Check sheet for the modelled part. Datum: model origin and axes. Units: mm. Face numbers are marked on the shaded views. A direction names the side the tool comes from. Coordinates: 2 decimals unless noted, no trailing zeros. Order: outer loops, then holes, each group sorted by start corner. A loop starts at its lowest first (then second) coordinate and runs counter-clockwise, first axis right, second up.
from build123d import *

# Parameters (mm, degrees)
SKETCH1_W           = 50
SKETCH1_H           = 25
BOSS_EXTRUDE1_DEPTH = 5
SKETCH2_W           = 45
SKETCH2_H           = 20
BOSS_EXTRUDE2_DEPTH = 40
SKETCH3_W           = 40
SKETCH3_H           = 12
CUT_EXTRUDE1_DEPTH  = 1
SKETCH4_W           = 6
SKETCH4_H           = 2
BOSS_EXTRUDE3_DEPTH = 1


with BuildPart() as part:
    # Sketch1 → Boss-Extrude1 (new body)
    with BuildSketch(Plane(origin=(0, 0, 0), x_dir=(1, 0, 0), z_dir=(0, 1, 0))):
        with Locations((25, 12.5)):
            Rectangle(SKETCH1_W, SKETCH1_H)
    extrude(amount=-BOSS_EXTRUDE1_DEPTH)

    # Sketch2 → Boss-Extrude2 (add)
    with BuildSketch(Plane.XZ.offset(5)):
        with Locations((25, -12.5)):
            Rectangle(SKETCH2_W, SKETCH2_H)
    extrude(amount=BOSS_EXTRUDE2_DEPTH)

    # Sketch3 → Cut-Extrude1 (cut)
    with BuildSketch(Plane(origin=(0, 0, 0), x_dir=(1, 0, 0), z_dir=(0, 1, 0))):
        with Locations((25, 16)):
            Rectangle(SKETCH3_W, SKETCH3_H)
    extrude(amount=-CUT_EXTRUDE1_DEPTH, mode=Mode.SUBTRACT)

    # Sketch4 → Boss-Extrude3 (add)
    with BuildSketch(Plane(origin=(0, 0, 0), x_dir=(1, 0, 0), z_dir=(0, 1, 0))):
        with Locations((42, 6)):
            Rectangle(SKETCH4_W, SKETCH4_H)
    extrude(amount=BOSS_EXTRUDE3_DEPTH)


solid = part.part
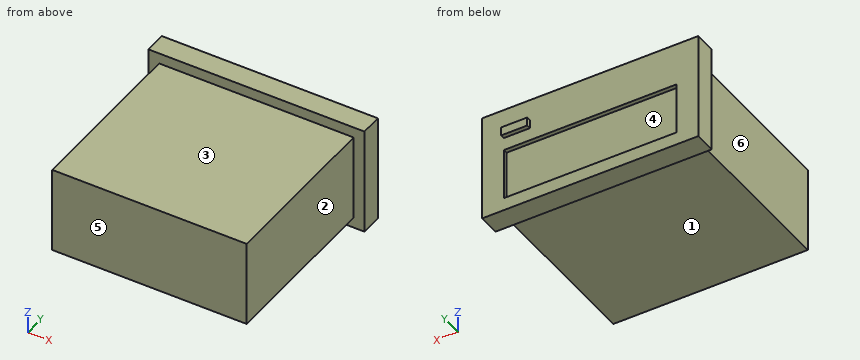
(1) Release check for a two-part mould opening along X. For the marked faces 4, 5 and 6 record: +X half, -X half, draft (parallel to the pull), parting line (faces both ways), or undercut.
Filled in:
face 4: undercut
face 5: draft
face 6: -X half
(2) Cross-section at A-A (x = 41). Enter the section's corners in (y, z), and give its area (3 significant figures).
Filled in:
outline: (-45, -22.5) - (-5, -22.5) - (-5, -25) - (0, -25) - (0, -22) - (-1, -22) - (-1, -10) - (0, -10) - (0, -7) - (1, -7) - (1, -5) - (0, -5) - (0, 0) - (-5, 0) - (-5, -2.5) - (-45, -2.5) - close
area: 915 mm2
(3) Cross-section at B-B (z = -16.5). Enter the section's corners in (x, y).
Filled in:
outline: (0, -5) - (2.5, -5) - (2.5, -45) - (47.5, -45) - (47.5, -5) - (50, -5) - (50, 0) - (45, 0) - (45, -1) - (5, -1) - (5, 0) - (0, 0) - close
(4) Cross-section at C-C (x = 21.5). Enter the section's corners in (y, z).
Filled in:
outline: (-45, -22.5) - (-5, -22.5) - (-5, -25) - (0, -25) - (0, -22) - (-1, -22) - (-1, -10) - (0, -10) - (0, 0) - (-5, 0) - (-5, -2.5) - (-45, -2.5) - close
(5) Go/stop test with flat-tipped pins: P1, Ø3.5, axis at x = 28.5, z = -17, coming from the +Y side; P2, Ø0.8, axis at x = 42.5, y = 0.5, coming from the -Z side; P3, Ø12, axis at x = 30, y = -20, coming from the +Z side. Record where each tip stops, or that it passes through.
Filled in:
P1: stops at y = -1
P2: stops at z = -7
P3: stops at z = -2.5
(6) Tool access check on the marked faces 1, 2 and 3. Record the directions out of +Z, -Z, +X, -X, +Y, -Y that give a thin tool (end or side, any length) a straight path to the whole face; none if there is none.
Filled in:
face 1: -Z, +X, -X, -Y
face 2: +Z, -Z, +X, -Y
face 3: +Z, +X, -X, -Y
(7) Thickness scan on probe 1 along X at (y, z) = (-39, -10); probe 2 along Z at (x, y) = (46, -6.5); probe 3 along Y at (x, z) = (42.5, -10.5). Record the ranges inside material, lowest first.
Filled in:
probe 1: x = 2.5 to 47.5
probe 2: z = -22.5 to -2.5
probe 3: y = -45 to -1
(8) Cross-section at D-D (y = -12). Enter the section's corners in (x, z).
Filled in:
outline: (2.5, -22.5) - (47.5, -22.5) - (47.5, -2.5) - (2.5, -2.5) - close
